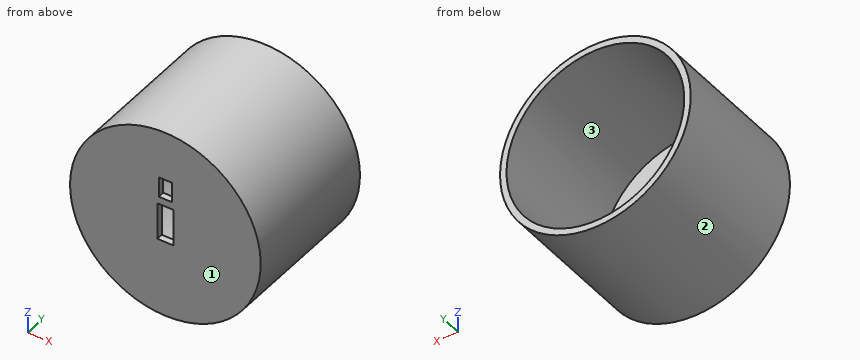
```python
from build123d import *

# Parameters (mm, degrees)
SKETCH1_R           = 118
BOSS_EXTRUDE1_DEPTH = 180
SKETCH3_R           = 110
CUT_EXTRUDE1_DEPTH  = 172
SKETCH6_W           = 19.77
SKETCH6_H           = 45.83
CUT_EXTRUDE2_DEPTH  = 240.649744419
SKETCH7_W           = 16.617647061
SKETCH7_H           = 25
CUT_EXTRUDE3_DEPTH  = 158


with BuildPart() as part:
    # Sketch1 → Boss-Extrude1 (new body)
    with BuildSketch(Plane(origin=(0, 0, 0), x_dir=(1, 0, 0), z_dir=(0, 1, 0))):
        with Locations(Location((0, 0, 0), (0, 0, 90))):
            Circle(SKETCH1_R)
    extrude(amount=BOSS_EXTRUDE1_DEPTH)

    # Sketch3 → Cut-Extrude1 (cut)
    with BuildSketch(Plane(origin=(0, 180, 0), x_dir=(1, 0, 0), z_dir=(0, 1, 0))):
        with Locations(Location((0, 0, 0), (0, 0, 270))):
            Circle(SKETCH3_R)
    extrude(amount=-CUT_EXTRUDE1_DEPTH, mode=Mode.SUBTRACT)

    # Sketch6 → Cut-Extrude2 (cut, through all)
    with BuildSketch(Plane(origin=(0, 8, 0), x_dir=(1, 0, 0), z_dir=(0, 1, 0))):
        Rectangle(SKETCH6_W, SKETCH6_H)
    extrude(amount=-CUT_EXTRUDE2_DEPTH, mode=Mode.SUBTRACT)

    # Sketch7 → Cut-Extrude3 (cut)
    with BuildSketch(Plane.XZ):
        with Locations((0.107153446, 44.591409708)):
            Rectangle(SKETCH7_W, SKETCH7_H)
    extrude(amount=-CUT_EXTRUDE3_DEPTH, mode=Mode.SUBTRACT)


solid = part.part
```
The model under review builds one solid part; all positions refer to its coordinate system, in mm. Face numbers are marked on the shaded views. Round coordinates to 2 decimals unless told otherwise and drop trailing zeros. Loops run counter-clockwise (first coordinate to the right, second up) from the corner with the lowest first, then second, coordinate; pieces in that order, holes last. Notation, with made-up numbers: M 28,47.25 L 40,47.25 A17 cw 40,79.25 Z; hole C 69.5,57.25 d4. An arc over 180 degrees is marked long. Answer as a JSON object with one key per item and string values.
(1) Take a section at C-C on y = 36. Give the boundary of the cut face in (x, z), and give its area (3 significant figures).
Resolved:
{"outline": "C 0,0 d236; hole C 0,0 d220", "area": "5,730 mm²"}
(2) Take a section at A-A on x = 0. Give the boundary of the cut face in (y, z) (3 decimals), and give its area (3 significant figures).
Resolved:
{"outline": "M 0,-118 L 180,-118 L 180,-110 L 8,-110 L 8,-22.915 L 0,-22.915 Z; M 0,22.915 L 8,22.915 L 8,32.091 L 0,32.091 Z; M 0,57.091 L 8,57.091 L 8,110 L 180,110 L 180,118 L 0,118 Z", "area": "4,070 mm²"}
(3) Draft analysis for pull direction X (two halves, no side actions). For the marked faces 1, 2 and 3, state which applies: released by +X, released by -X, zero draft, split by the parting line, or undercut.
Resolved:
{"face 1": "zero draft", "face 2": "split by the parting line", "face 3": "undercut"}
(4) Take a section at D-D on z = 99.5. Give the boundary of the cut face in (x, y).
Resolved:
{"outline": "M -63.43,0 L 63.43,0 L 63.43,180 L 46.9,180 L 46.9,8 L -46.9,8 L -46.9,180 L -63.43,180 Z"}
(5) To check wall thickness, follow line 1 along X through (y, z) = (96.5, 0); line 2 along Y through (x, z) = (24.5, 6); line 3 along X through (y, z) = (64, -95.5). State the ranges of each line that lie inside material, in increasing order.
Resolved:
{"line 1": "-118 to -110, 110 to 118", "line 2": "0 to 8", "line 3": "-69.31 to -54.59, 54.59 to 69.31"}
(6) Take a section at B-B on z = 0. Give the boundary of the cut face in (x, y) (3 decimals).
Resolved:
{"outline": "M -118,0 L -9.885,0 L -9.885,8 L -110,8 L -110,180 L -118,180 Z; M 9.885,0 L 118,0 L 118,180 L 110,180 L 110,8 L 9.885,8 Z"}
(7) Clearance check with flat-ended pins moving along their axes: P1, Ø9, axis at y = 5, z = 41.5, coming from the +X side; P2, Ø1.5, axis at x = -10.5, y = 30, coming from the -Z side; P3, Ø6.5, axis at y = 3.5, z = 47, coming from the -X side. State where each tip first meets the part, or that it passes through.
Resolved:
{"P1": "x = 112.05", "P2": "z = -117.6", "P3": "x = -109.59"}
